from build123d import *

# Parameters (mm, degrees)
BOSS_EXTRUDE1_DEPTH = 375
FILLET1_R           = 100
FILLET2_R           = 100


with BuildPart() as part:
    # Sketch1 → Boss-Extrude1 (new body)
    with BuildSketch(Plane(origin=(0, 0, 0), x_dir=(1, 0, 0), z_dir=(0, 1, 0))):
        with BuildLine():
            ThreePointArc((-611.4919693133057, 0), (-432.39011814255474, -432.3901181425547), (-3.744e-14, -611.4919693133057))
            Line((0, -611.4919693133057), (0, -187.5))
            ThreePointArc((-1.86631e-12, -187.5), (-132.58252147247833, -132.58252147247697), (-187.5, 2.296e-14))
            Line((-187.5, 0), (-611.4919693133057, 0))
        make_face()
        with BuildLine():
            Line((0, -187.5), (0, -611.4919693133057))
            ThreePointArc((-3.744e-14, -611.4919693133057), (432.3901181425547, -432.39011814255474), (611.4919693133057, -7.489e-14))
            Line((611.4919693133057, 0), (187.5, 0))
            ThreePointArc((187.5, -4.592e-14), (132.58252147247705, -132.58252147247828), (-1.86631e-12, -187.5))
        make_face()
        with BuildLine():
            Line((187.5, 0), (611.4919693133057, 0))
            ThreePointArc((611.4919693133056, -2.2737e-13), (335.12599508158894, 243.9066567186602), (187.9999999999999, 581.8749251640463))
            ThreePointArc((188, 581.8749251640465), (95.15929973489084, 604.0423298152456), (0, 611.4919693133056))
            Line((0, 611.4919693133057), (0, 468.44559362451025))
            ThreePointArc((2.9354e-13, 468.44559362451025), (68.16635262601869, 442.2325840672666), (96.6892055692424, 375))
            ThreePointArc((96.6892055692424, 375), (68.16635262601865, 307.76741593273334), (2.7045e-13, 281.55440637548975))
            Line((0, 281.55440637548975), (0, 187.5))
            ThreePointArc((-1.90365e-12, 187.5), (132.58252147247697, 132.58252147247833), (187.5, 0))
        make_face()
        with BuildLine():
            ThreePointArc((-188, 581.8749251640467), (-335.1259950815888, 243.90665671866032), (-611.4919693133057, 0))
            Line((-611.4919693133057, 0), (-187.5, 0))
            ThreePointArc((-187.5, 2.296e-14), (-132.5825214724783, 132.58252147247703), (-1.90365e-12, 187.5))
            Line((0, 187.5), (0, 281.55440637548975))
            ThreePointArc((2.7045e-13, 281.55440637548975), (-90.3107944307576, 375), (2.9354e-13, 468.44559362451025))
            Line((0, 468.44559362451025), (0, 611.4919693133057))
            ThreePointArc((0, 611.4919693133056), (-95.15929973489085, 604.0423298152457), (-188.00000000000003, 581.8749251640465))
        make_face()
    extrude(amount=BOSS_EXTRUDE1_DEPTH)

    # Fillet1
    fillet1_edges = [part.edges().sort_by_distance(p)[0] for p in [
        (-335.12599508158894, 375, -243.90665671866043),
        (-3.111e-14, 375, 611.4919693133057),
        (335.12599508158894, 375, -243.9066567186602),
        (-7.11e-15, 375, -611.4919693133056),
    ]]
    fillet(fillet1_edges, radius=FILLET1_R)

    # Fillet2
    fillet2_edges = [part.edges().sort_by_distance(p)[0] for p in [
        (-1.027e-14, 0, 611.4919693133057),
        (-335.12599508158894, 0, -243.90665671866043),
        (-2.132e-14, 0, -611.4919693133056),
        (335.12599508158894, 0, -243.9066567186602),
    ]]
    fillet(fillet2_edges, radius=FILLET2_R)


solid = part.part
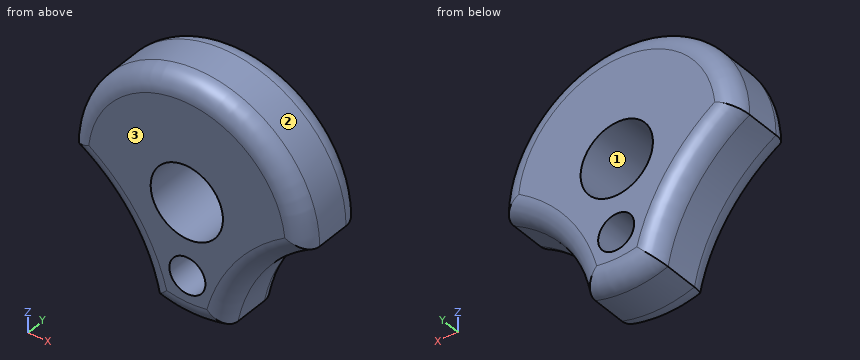
The model under review builds one solid part; all positions refer to its coordinate system, in mm. Face numbers are marked on the shaded views. Round coordinates to 2 decimals unless told otherwise and drop trailing zeros. Write each loop counter-clockwise with the first axis right and the second up, starting at its lowest first coordinate (ties: lowest second). Pieces come first, ordered by that corner, then holes. Notation, with made-up numbers: M -29.5,-2 L -12.5,-2 A21 ccw -12.5,11 Z; hole C 48,64 d5. An arc over 180 degrees is marked long. Use a Markdown table: item, result. Add a question column.
Q1. The part is to be moulded in two halves that separate along X. For the marked faces 1, 2 and 3, say which applies: pulls with the +X half, pulls with the -X half, needs draft (parallel to the pull), parting line crosses it, or undercut.
Q2. Insertion check: pin 1 (8 mm diameter, centred on y = 44, z = 89, fed in from +X); pin 2 (4 mm diameter, centred on x = 266.5, y = 179, fed in from +Z); pin 3 (6 mm diameter, centred on x = 242.5, y = 79, fed in from +Z). Each pin has a flat end and moves straight along its axis. Give the tip position at first contact, or say it passes through.
Q3. We need section A-A, the plane y = 302. State the section outline as (x, z) points, plus the area to 3 significant figures.
Q4. To check wall thickness, follow line 1 (X direction, y = 238, z = 0); line 2 (Z direction, x = -50, y = 80.5); line 3 (Z direction, x = 21, y = 225.5). State the ranges of each line that lie inside material, in increasing order.
Q5. We need section C-C, the plane y = 180.5. State the section outline as (x, z) points.
Q6. We need section B-B, the plane x = 0. Count the separate pieces of the cut face and the enclosed holes in it, plus the area to 3 significant figures.
Findings below:
| question | item | result |
|---|---|---|
| 1 | face 1 | undercut |
| 1 | face 2 | parting line crosses it |
| 1 | face 3 | needs draft |
| 2 | pin 1 | stops at x = 590.31 |
| 2 | pin 2 | stops at z = 551.33 |
| 2 | pin 3 | stops at z = 560.38 |
| 3 | outline | M -607.77,2.19 A853.71 cw -184.78,-579.01 A607.78 ccw 184.78,-579.01 A853.71 cw 607.77,2.19 A607.78 ccw Z; hole C 0,0 d375; hole C 3.19,-375 d187 |
| 3 | area | 831,000 mm² |
| 4 | line 1 | x = -611.49 to -187.5, 187.5 to 611.49 |
| 4 | line 2 | z = -607.52 to -451.9, -298.1 to -180.71, 180.71 to 607.52 |
| 4 | line 3 | z = -611.13 to -466.79, -283.21 to -186.32, 186.32 to 611.13 |
| 5 | outline | M -611.49,0 A850 cw -188,-581.87 A611.49 ccw 188,-581.87 A850 cw 611.49,0 A611.49 ccw Z; hole C 0,0 d375; hole C 3.19,-375 d187 |
| 6 | separate pieces | 3 |
| 6 | enclosed holes | 0 |
| 6 | area | 239,000 mm² |
